from build123d import *

# Parameters (mm, degrees)
F0_W     = 33.974414
F0_H     = 20.238973
F1_DEPTH = 25.4
F3_DEPTH = 12.7


with BuildPart() as f1:
    # F0 (on Front) → F1 (new body)
    with BuildSketch(Plane.XZ):
        with Locations((-1.508936, 12.108095)):
            Rectangle(F0_W, F0_H)
    extrude(amount=F1_DEPTH)

    # F2 (on Right) → F3 (cut, symmetric)
    with BuildSketch(Plane.YZ):
        Polygon((-31.785678, 39.70434), (-39.439067, 30.098028), (11.018346, -7.099656), (15.880866, 4.716209), (-1.683568, 11.944407), (7.317314, 17.191587), (0.589001, 25.465947), (-6.135374, 17.646428), align=None)
    extrude(amount=F3_DEPTH, both=True, mode=Mode.SUBTRACT)


solid = f1.part
Source: CAD feature listing. Evaluate the final solid. Frame: model axes, mm. A direction names the side the tool comes from. Coordinates: 2 decimals unless noted, no trailing zeros. Loops run counter-clockwise (first coordinate to the right, second up) from the corner with the lowest first, then second, coordinate; pieces in that order, holes last. Notation, with made-up numbers: (77, 45) - (111, 45) arc R9 ccw to (111, 60) - close; hole circle Ø6 at (-7.75, 49.25). An arc over 180 degrees is marked (long way). Return JSON: item names as keys, results as strings.
Q1. Contact query for flat-ended pins moving along their axis: P1, Ø5, axis at x = 1.5, y = -16, coming from the +Z side; P2, Ø1, axis at x = -6, z = 4.5, coming from the +Y side. Output: stop coordinate, or through.
Results:
{"P1": "z = 14.66", "P2": "y = -4.04"}
Q2. Material intervals for line 1 along X through (y, z) = (-6.25, 11); line 2 along Z through (x, y) = (7, -3.5); line 3 along Z through (x, y) = (11, -8), sorted ascending.
Results:
{"line 1": "-18.5 to -12.7, 12.7 to 15.48", "line 2": "1.99 to 3.6, 20.71 to 22.23", "line 3": "1.99 to 6.92, 19.25 to 22.23"}
Q3. Section C-C, the plane z = 4. Return loops of the section in (x, y), plus the area to 3 significant figures.
Results:
{"outline": "(-18.5, -25.4) - (15.48, -25.4) - (15.48, 0) - (12.7, 0) - (12.7, -4.04) - (-12.7, -4.04) - (-12.7, 0) - (-18.5, 0) - close", "area": "760 mm2"}
Q4. Section D-D, the plane y = -23.25. Return loops of the section in (x, z), plus the area to 3 significant figures.
Results:
{"outline": "(-18.5, 1.99) - (15.48, 1.99) - (15.48, 22.23) - (12.7, 22.23) - (12.7, 18.16) - (-12.7, 18.16) - (-12.7, 22.23) - (-18.5, 22.23) - close", "area": "584 mm2"}
Q5. Access query for faces 5 (the flat face through (0.178, -8.762, 19.905)), 6 (the flat face through (0.2, -0.9, 12.4)), 7 (the flat face through (-6, 0, 12)). Directions: +Z, -Z, +X, -X, +Y, -Y. A direction counts if a zero-diameter tool reaches every point of the face in a straight line with its end or side. Return the directions, or none.
Results:
{"face 5": "none", "face 6": "+Z", "face 7": "+Z, -Z, +X, -X, +Y"}
Q6. Section B-B, the plane y = -9. Return loops of the section in (x, z), plus the area to 3 significant figures.
Results:
{"outline": "(-18.5, 1.99) - (15.48, 1.99) - (15.48, 22.23) - (-18.5, 22.23) - close; hole (-12.7, 7.66) - (12.7, 7.66) - (12.7, 20.11) - (-12.7, 20.11) - close", "area": "371 mm2"}
Q7. Section A-A, the plane x = -0.5. Return loops of the section in (y, z), plus the area to 3 significant figures.
Results:
{"outline": "(-25.4, 1.99) - (-1.31, 1.99) - (-25.4, 19.75) - close; (-11.46, 22.23) - (-6.14, 17.65) - (-2.2, 22.23) - close; (-1.68, 11.94) - (0, 11.25) - (0, 12.93) - close", "area": "237 mm2"}
Q8. Mould query, pull axis Y, two halves, no side actions, for faces 1 (the flat face through (-2, -25.4, 12)), 2 (the flat face through (15.478, -13, 12)), 3 (the flat face through (0.178, -4.138, 19.969)), 4 (the flat face through (-12.7, -10, 14)). Classes: released by +Y, released by -Y, zero draft, split by the parting line, or undercut.
Results:
{"face 1": "released by -Y", "face 2": "zero draft", "face 3": "released by +Y", "face 4": "undercut"}
